from build123d import *

# Parameters (mm, degrees)
SKETCH1_W                             = 154.05
SKETCH1_H                             = 40
BOSS_EXTRUDE1_DEPTH                   = 6.35
SKETCH2_W                             = 6.35
SKETCH2_H                             = 40
BOSS_EXTRUDE2_DEPTH                   = 40
FILLET1_R                             = 6.35
TAP_DRILL_FOR_M8_HELICOIL1_AT_2_COUNT = 2
TAP_DRILL_FOR_M8_HELICOIL1_AT_2_PITCH = 13.884315024
FILLET1_OF_MIRROR1_R                  = 6.35
SKETCH6_R                             = 2.5
CUT_EXTRUDE1_DEPTH                    = 40


with BuildPart() as part:
    # Sketch1 → Boss-Extrude1 (new body)
    with BuildSketch(Plane(origin=(0, 0, 0), x_dir=(1, 0, 0), z_dir=(0, 1, 0))):
        with Locations((-77.025, 20)):
            Rectangle(SKETCH1_W, SKETCH1_H)
    boss_extrude1 = extrude(amount=BOSS_EXTRUDE1_DEPTH)

    # Sketch2 → Boss-Extrude2 (add)
    with BuildSketch(Plane(origin=(0, 6.35, 0), x_dir=(1, 0, 0), z_dir=(0, 1, 0))):
        with Locations((-3.175, 20)):
            Rectangle(SKETCH2_W, SKETCH2_H)
    boss_extrude2 = extrude(amount=BOSS_EXTRUDE2_DEPTH)

    # Fillet1
    fillet1_edges = [part.edges().sort_by_distance(p)[0] for p in [
        (-6.35, 6.35, -20),
        (0, 0, -20),
    ]]
    fillet(fillet1_edges, radius=FILLET1_R)

    # Sketch5 → Tap Drill for M8 Helicoil1 (revolve, cut)
    with BuildSketch(Plane(origin=(-6.35, 36.467, -20), x_dir=(0, 0, 1), z_dir=(0, 1, 0))):
        Polygon((0, 0), (0, 6.35), (4.125, 6.35), (4.125, 0.025), (4.15, 0), align=None)
    tap_drill_for_m8_helicoil1 = revolve(axis=Axis((-12.7, 36.467, -20), (1, 0, 0)), mode=Mode.SUBTRACT)

    # Tap Drill for M8 Helicoil1 at 2: Tap Drill for M8 Helicoil1 ×2
    with Locations(*[Vector(0, -0.9999773107839142, -0.006736313336781501) * (i * TAP_DRILL_FOR_M8_HELICOIL1_AT_2_PITCH) for i in range(1, TAP_DRILL_FOR_M8_HELICOIL1_AT_2_COUNT)]):
        add(tap_drill_for_m8_helicoil1, mode=Mode.SUBTRACT)

    # Mirror1: Boss-Extrude1, Boss-Extrude2, Tap Drill for M8 Helicoil1 across plane
    add(boss_extrude1.mirror(Plane.ZY.offset(80.2)))
    add(boss_extrude2.mirror(Plane.ZY.offset(80.2)))
    add(tap_drill_for_m8_helicoil1.mirror(Plane.ZY.offset(80.2)), mode=Mode.SUBTRACT)

    # Mirror1 copy 1 sketch → Mirror1 copy 1 (revolve, cut)
    with BuildSketch(Plane(origin=(-154.05, 22.583, -20.093529096), x_dir=(0, 0, 1), z_dir=(0, 1, 0))):
        Polygon((0, 0), (0, -6.35), (4.125, -6.35), (4.125, -0.025), (4.15, 0), align=None)
    revolve(axis=Axis((-147.7, 22.583, -20.093529096), (1, 0, 0)), mode=Mode.SUBTRACT)

    # Fillet1 of Mirror1
    fillet1_of_mirror1_edges = [part.edges().sort_by_distance(p)[0] for p in [
        (-154.05, 6.35, -20),
        (-160.4, 0, -20),
    ]]
    fillet(fillet1_of_mirror1_edges, radius=FILLET1_OF_MIRROR1_R)

    # Sketch6 → Cut-Extrude1 (cut)
    with BuildSketch(Plane(origin=(0, 6.35, 0), x_dir=(1, 0, 0), z_dir=(0, 1, 0))):
        with Locations(Location((-98.2, 20, 0), (0, 0, 270))):
            Circle(SKETCH6_R)
        with Locations(Location((-62.2, 20, 0), (0, 0, 270))):
            Circle(SKETCH6_R)
    extrude(amount=-CUT_EXTRUDE1_DEPTH, mode=Mode.SUBTRACT)


solid = part.part
Input: part model. Units: mm. Frame: model coordinates. A direction names the side the tool comes from. Coordinates: 2 decimals unless noted, no trailing zeros. Loops run counter-clockwise (first coordinate to the right, second up) from the corner with the lowest first, then second, coordinate; pieces in that order, holes last. Notation, with made-up numbers: (75, -8.75) -> (110, -8.75) arc R23 cw to (110, 0.25) -> close; hole circle Ø4 at (14, 59.5). An arc over 180 degrees is marked (long way). One line per item, written item: value.
(1) Pin query (flat end, axial travel): pin 1 Ø13 at (y, z) = (22.58, -20.09) entering from +X; pin 2 Ø10 at (x, z) = (-139, -4.5) entering from +Y. Return the tip coordinate at first contact, or that it passes through.
Answer below:
pin 1: stops at x = 0
pin 2: stops at y = 6.35
(2) Cut plane A-A (x = -62.2). Output: boundary loops of the cut face in (y, z), then the cut area to 3 significant figures.
Answer below:
outline: (0, -40) -> (6.35, -40) -> (6.35, -22.5) -> (0, -22.5) -> close; (0, -17.5) -> (6.35, -17.5) -> (6.35, 0) -> (0, 0) -> close
area: 222 mm2
(3) Ray query, line 1 along X through (y, z) = (36.5, -29.5); line 2 along Y through (x, z) = (-3.25, -20). Return the intervals inside material, ascending.
Answer below:
line 1: x = -160.4 to -154.05, -6.35 to 0
line 2: y = 0.81 to 18.46, 26.71 to 32.34, 40.59 to 46.35
(4) Cut plane C-C (z = -3). Output: boundary loops of the cut face in (x, y), then the cut area to 3 significant figures.
Answer below:
outline: (-160.4, 6.35) arc R6.35 ccw to (-154.05, 0) -> (-6.35, 0) arc R6.35 ccw to (0, 6.35) -> (0, 46.35) -> (-6.35, 46.35) -> (-6.35, 12.7) arc R6.35 cw to (-12.7, 6.35) -> (-147.7, 6.35) arc R6.35 cw to (-154.05, 12.7) -> (-154.05, 46.35) -> (-160.4, 46.35) -> close
area: 1,530 mm2
(5) Set-up query: faces 4 (the face through (-81, 6.35, -20)), 5 (the face through (-81, 0, -20)). Return all of +Z, -Z, +X, -X, +Y, -Y with unobstructed straight access to the full face (end or side cutting, diameter ignored); none if empty.
Answer below:
face 4: +Z, -Z, +Y
face 5: +Z, -Z, +X, -X, -Y
(6) Cut plane D-D (x = -94). Output: boundary loops of the cut face in (y, z).
Answer below:
outline: (0, -40) -> (6.35, -40) -> (6.35, 0) -> (0, 0) -> close
(7) Cut plane B-B (y = 14.5). Output: boundary loops of the cut face in (x, z), then the cut area to 3 significant figures.
Answer below:
outline: (-160.4, -40) -> (-154.05, -40) -> (-154.05, 0) -> (-160.4, 0) -> close; (-6.35, -40) -> (0, -40) -> (0, 0) -> (-6.35, 0) -> close
area: 508 mm2
(8) Draft query along Z for faces 1 (the face through (-80, 6, 0)), 2 (the face through (-59.72, 3.22, -20.33)), 3 (the face through (-8.16, 8.26, -20.28)). Return one class per face: pulls with the +Z half, pulls with the -Z half, needs draft (parallel to the pull), parting line crosses it, or undercut.
Answer below:
face 1: pulls with the +Z half
face 2: undercut
face 3: needs draft
